Geometry check sheet. Reference: the model listing, model coordinates, mm. A direction names the side the tool comes from. Round coordinates to 2 decimals unless told otherwise and drop trailing zeros. Order: outer loops, then holes, each group sorted by start corner. A loop starts at its lowest first (then second) coordinate and runs counter-clockwise, first axis right, second up. Notation, with made-up numbers: M -30,-33 L 19,-33 A22 ccw 19,-20 Z; hole C -34,75.25 d1. An arc over 180 degrees is marked long. Return JSON: item names as keys, results as strings. Group by question number.
```python
from build123d import *

# Parameters (mm, degrees)
SKETCH_1_R      = 1.35
EXTRUDE_1_DEPTH = 2.35
SKETCH_3_R      = 0.4
SKETCH_2_R      = 0.4


with BuildPart() as part:
    # Эскиз1 → Бобышка-Вытянуть1 (new, symmetric)
    with BuildSketch(Plane.XY):
        Circle(SKETCH_1_R)
    extrude(amount=EXTRUDE_1_DEPTH, both=True)

    # По траектории1: sweep along a path in Эскиз5
    with BuildLine(Plane(origin=(0, 0, 0), x_dir=(0, 0, -1), z_dir=(1, 0, 0))) as sweep_1_path:
        Line((2.35, 0), (3, 0))
        ThreePointArc((3, 0), (3.707106781, -0.292893219), (4, -1))
        Line((4, -1), (4, -4.35))
    # Эскиз3 → По траектории1 (sweep)
    with BuildSketch(Plane(origin=(0, 0, -2.35), x_dir=(-1, 0, 0), z_dir=(0, 0, -1))):
        Circle(SKETCH_3_R)
    sweep(path=sweep_1_path.line)

    # По траектории2: sweep along a path in Эскиз6
    with BuildLine(Plane(origin=(0, 0, 0), x_dir=(0, 0, -1), z_dir=(1, 0, 0))) as sweep_2_path:
        Line((-2.35, 0), (-3, 0))
        ThreePointArc((-3, 0), (-3.707106781, -0.292893219), (-4, -1))
        Line((-4, -1), (-4, -4.35))
    # Эскиз2 → По траектории2 (sweep)
    with BuildSketch(Plane.XY.offset(2.35)):
        Circle(SKETCH_2_R)
    sweep(path=sweep_2_path.line)


solid = part.part
```
Q1. Section check D-D on x = 0.9. Record the cut outline in (y, z), plus the area to 3 significant figures.
Q2. Set-up check for faces 1 (the face through (1, 0, 2.35)), 2 (the face through (0.052, -2.698, -4.397)): record each of +Z, -Z, +X, -X, +Y, -Y from which the full face is reachable in a straight line by a thin tool's end or side.
Q3. Section check C-C on z = 2.5. Record the cut outline in (x, y).
Q4. Section check A-A on x = 0. Record the cut outline in (y, z), plus the area to 3 significant figures.
Q5. Material ranges on line 1 along Z through (x, y) = (-0.5, 0.1); line 2 along X through (y, z) = (0.8, 1.75); line 3 along Y through (x, z) = (-0.7, -2.25), recorded low to high.
Q6. Section check B-B on y = -2.1. Record the cut outline in (x, z).
Q7. Depth check by flat-ended pin: pin 1 Ø1.5 at (x, z) = (0, 0) entering from -Y; pin 2 Ø3 at (y, z) = (-2.5, 2) entering from -X; pin 3 Ø0.8 at (x, y) = (0, -0.5) entering from -Z. Enter the tip coordinate at first touch or a pass-through.
Geometry check:
{
 "1": {"outline": "M -1.01,-2.35 L 1.01,-2.35 L 1.01,2.35 L -1.01,2.35 Z", "area": "9.46 mm^2"},
 "2": {"face 1": "none", "face 2": "-Y"},
 "3": {"outline": "C 0,0 d0.8"},
 "4": {"outline": "M -4.35,-4.4 L -1,-4.4 A1.4 ccw 0.4,-3 L 0.4,-2.35 L 1.35,-2.35 L 1.35,2.35 L 0.4,2.35 L 0.4,3 A1.4 ccw -1,4.4 L -4.35,4.4 L -4.35,3.6 L -1,3.6 A0.6 cw -0.4,3 L -0.4,2.35 L -1.35,2.35 L -1.35,-2.35 L -0.4,-2.35 L -0.4,-3 A0.6 cw -1,-3.6 L -4.35,-3.6 Z", "area": "21.6 mm^2"},
 "5": {"line 1": "z = -2.35 to 2.35", "line 2": "x = -1.09 to 1.09", "line 3": "y = -1.15 to 1.15"},
 "6": {"outline": "C 0,-4 d0.8; C 0,4 d0.8"},
 "7": {"pin 1": "stops at y = -1.35", "pin 2": "stops at x = -0.91", "pin 3": "stops at z = -4.4"}
}
